```python
from build123d import *

# Parameters (mm, degrees)
CYLINDER009_R     = 37
CYLINDER009_DEPTH = 2.8
CYLINDER010_R     = 45
CYLINDER010_DEPTH = 2.8
SKETCH005_R       = 1.8
POCKET003_DEPTH   = 5
PAD_DEPTH         = 3
CHAMFER_SIZE      = 1
CHAMFER001_SIZE   = 1
CHAMFER002_SIZE   = 1
CHAMFER003_SIZE   = 1


with BuildPart() as cylinder009:
    # Cylinder009 → Cylinder009 (new body)
    with BuildSketch(Plane.XY.offset(83)):
        Circle(CYLINDER009_R)
    extrude(amount=CYLINDER009_DEPTH)


with BuildPart() as chamfer003:
    # Cylinder010 → Cylinder010 (new body)
    with BuildSketch(Plane.XY.offset(83)):
        Circle(CYLINDER010_R)
    extrude(amount=CYLINDER010_DEPTH)

    # Cut008: cut Cylinder009
    add(cylinder009.part, mode=Mode.SUBTRACT)

    # Sketch005 → Pocket003 (cut)
    with BuildSketch(Plane.XY.offset(85.8)):
        with Locations((10.92856, 38.840008)):
            Circle(SKETCH005_R)
        with Locations((40.444542, -6.343234)):
            Circle(SKETCH005_R)
        with Locations((-10.194257, -38.936714)):
            Circle(SKETCH005_R)
        with Locations((-39.850128, 8.065043)):
            Circle(SKETCH005_R)
    extrude(amount=-POCKET003_DEPTH, mode=Mode.SUBTRACT)

    # Sketch006 → Pad (new body)
    with BuildSketch(Plane.XY.offset(85.8)):
        with BuildLine():
            ThreePointArc((32.2, 0), (30.678353, 9.781545), (26.257228, 18.638615))
            Line((26.257228, 18.638615), (35.943074, 27.075735))
            ThreePointArc((45, 0), (42.675744, 14.275182), (35.943074, 27.075735))
            Line((32.2, 0), (45, 0))
        make_face()
        with BuildLine():
            ThreePointArc((-32.2, 0), (-30.108619, -11.415388), (-24.106144, -21.347923))
            Line((-24.106144, -21.347923), (-34.666195, -28.692419))
            ThreePointArc((-45, 0), (-42.337801, -15.248299), (-34.666195, -28.692419))
            Line((-32.2, 0), (-45, 0))
        make_face()
    extrude(amount=PAD_DEPTH)

    # Chamfer
    chamfer_edges = [chamfer003.edges().sort_by_distance(p)[0] for p in [
        (-38.6, 0, 88.8),
    ]]
    chamfer(chamfer_edges, length=CHAMFER_SIZE)

    # Chamfer001
    chamfer001_edges = [chamfer003.edges().sort_by_distance(p)[0] for p in [
        (-29.38617, -25.020171, 88.8),
    ]]
    chamfer(chamfer001_edges, length=CHAMFER001_SIZE)

    # Chamfer002
    chamfer002_edges = [chamfer003.edges().sort_by_distance(p)[0] for p in [
        (31.100151, 22.857175, 88.8),
    ]]
    chamfer(chamfer002_edges, length=CHAMFER002_SIZE)

    # Chamfer003
    chamfer003_edges = [chamfer003.edges().sort_by_distance(p)[0] for p in [
        (38.6, 0, 88.8),
    ]]
    chamfer(chamfer003_edges, length=CHAMFER003_SIZE)


solid = chamfer003.part
```
CAD build for the part. Positions are in the model's coordinates, mm. A direction names the side the tool comes from. Give positions to 0.01 mm unless a question says otherwise; leave off trailing zeros. Write each loop counter-clockwise with the first axis right and the second up, starting at its lowest first coordinate (ties: lowest second). Pieces come first, ordered by that corner, then holes. Notation, with made-up numbers: (-40, 65.25) -> (6, 65.25) arc R22 cw to (6, 99.25) -> close; hole circle Ø6 at (77.5, -30). An arc over 180 degrees is marked (long way). Write each question's results on one line, items separated by ' | '.
1. Cut at C-C, the plane y = 16.5. Write the cut outline in (x, z).
Geometry check:
outline: (-41.87, 83) -> (-33.12, 83) -> (-33.12, 85.8) -> (-41.87, 85.8) -> close; (27.65, 85.8) -> (33.12, 85.8) -> (33.12, 83) -> (41.87, 83) -> (41.87, 88.8) -> (27.65, 88.8) -> close
2. Wall check: probe 1 along Y at (x, z) = (0, 83.8); probe 2 along Y at (x, z) = (-11.5, 84.9). Give the ranges that are in metal, low to high. Write a range as [from, to].
Geometry check:
probe 1: [-45, -37], [37, 45] | probe 2: [-43.51, -40.18], [-37.7, -35.17], [35.17, 43.51]
3. Cut at A-A, the plane x = 0. Write the cut outline in (y, z), then the cut area to 3 significant figures.
Geometry check:
outline: (-45, 83) -> (-37, 83) -> (-37, 85.8) -> (-45, 85.8) -> close; (37, 83) -> (45, 83) -> (45, 85.8) -> (37, 85.8) -> close | area: 44.8 mm²
4. Drop flat-ended pins along their axis: P1, Ø2, axis at y = 27, z = 84, coming from the +X side; P2, Ø1.5, axis at x = 7, z = 87, coming from the -Y side; P3, Ø1.6, axis at x = 39.5, z = 87, coming from the -Y side; P4, Ø6, axis at x = -39.85, y = 8.07, coming from the +Z side. Give the stop position or say it passes through.
Geometry check:
P1: x = 36.73 | P2: through | P3: y = 0 | P4: z = 85.8
5. Which spindle directions (+Z, -Z, +X, -X, +Y, -Y) get a long thin tool onto all of the face, cutting with end or side? Do faces 1 (the cylindrical face through (42.74, 14.08, 87.28)), 2 (the cylindrical face through (-8.02, -36.12, 84.38)), 3 (the flat face through (-39, 0, 87)), 4 (the flat face through (39, 0, 87)). Say none if no direction does.
Geometry check:
face 1: +Z, -Z, +X, +Y | face 2: -Z | face 3: +Z, -X, +Y | face 4: +Z, +X, -Y
6. Cut at D-D, the plane z = 84.8. Write the cut outline in (x, y).
Geometry check:
outline: circle Ø90 at (0, 0); hole circle Ø3.6 at (-39.85, 8.07); hole circle Ø74 at (0, 0); hole circle Ø3.6 at (-10.19, -38.94); hole circle Ø3.6 at (10.93, 38.84); hole circle Ø3.6 at (40.44, -6.34)
7. Cut at B-B, the plane x = -26.5. Write the cut outline in (y, z), then the cut area to 3 significant figures.
Geometry check:
outline: (-36.37, 83) -> (-25.82, 83) -> (-25.82, 85.8) -> (-36.37, 85.8) -> close; (-23.01, 85.8) -> (-18.29, 85.8) -> (-18.29, 88.8) -> (-21.79, 88.8) -> (-23.01, 87.8) -> close; (25.82, 83) -> (36.37, 83) -> (36.37, 85.8) -> (25.82, 85.8) -> close | area: 72.6 mm²
